Geometry: see drawing. Coordinates: mm, zero at the bounding-box minimum. A direction names the side the tool comes from. Coordinates: 2 decimals unless noted, no trailing zeros. Order: outer loops, then holes, each group sorted by start corner. A loop starts at its lowest first (then second) coordinate and runs counter-clockwise, first axis right, second up.
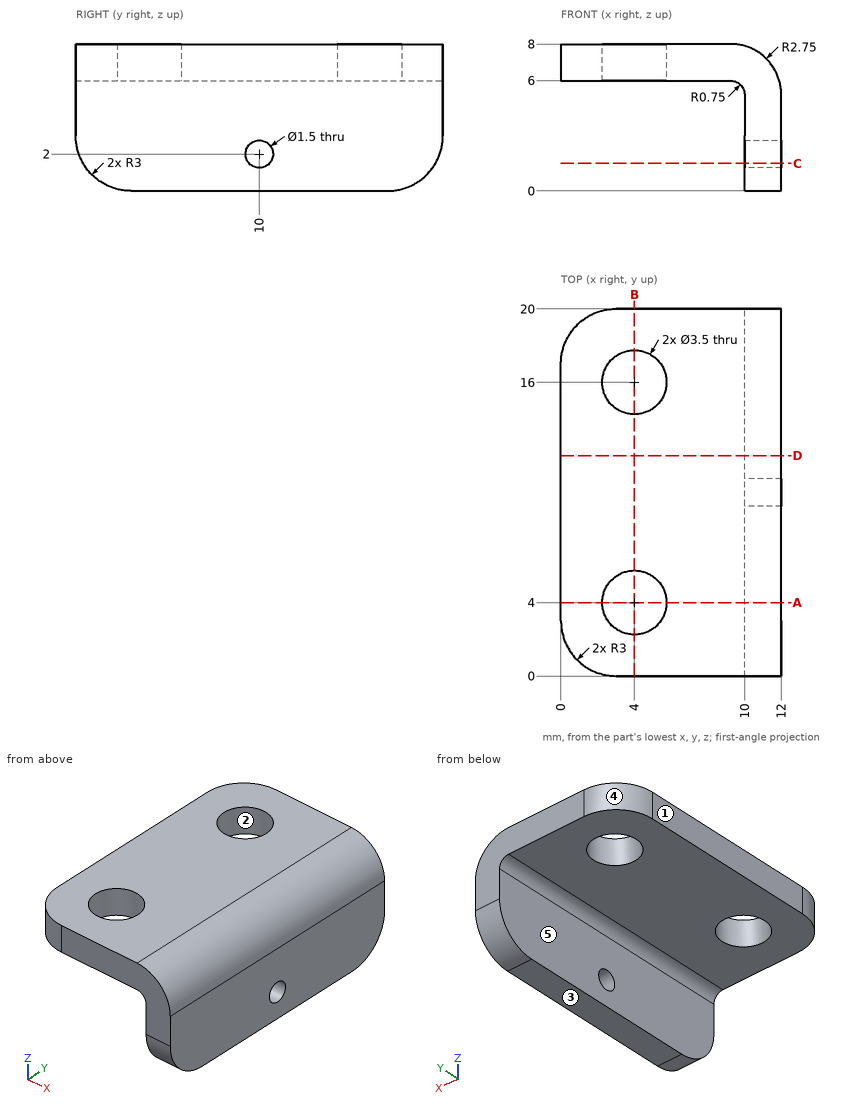
Item 1: Cut plane B-B on x = 4. Return loops of the section in (y, z).
Response values:
outline: (0, 6) - (2.25, 6) - (2.25, 8) - (0, 8) - close; (5.75, 6) - (14.25, 6) - (14.25, 8) - (5.75, 8) - close; (17.75, 6) - (20, 6) - (20, 8) - (17.75, 8) - close
Item 2: Access query for the marked faces 4 and 5. Directions: +Z, -Z, +X, -X, +Y, -Y. A direction counts if a zero-diameter tool reaches every point of the face in a straight line with its end or side. Return the directions, or none.
Response values:
face 4: +Z, -Z, -X, +Y
face 5: -Z, -X, +Y, -Y
Item 3: Cut plane A-A on y = 4. Return loops of the section in (x, z), then the cut area to 3 significant figures.
Response values:
outline: (0, 6) - (2.25, 6) - (2.25, 8) - (0, 8) - close; (5.75, 6) - (9.25, 6) arc R0.75 cw to (10, 5.25) - (10, 0) - (12, 0) - (12, 5.25) arc R2.75 ccw to (9.25, 8) - (5.75, 8) - close
area: 27.5 mm2
Item 4: Cut plane D-D on y = 12. Return loops of the section in (x, z), then the cut area to 3 significant figures.
Response values:
outline: (0, 6) - (9.25, 6) arc R0.75 cw to (10, 5.25) - (10, 0) - (12, 0) - (12, 5.25) arc R2.75 ccw to (9.25, 8) - (0, 8) - close
area: 34.5 mm2
Item 5: Draft query along X for the marked faces 1, 2 and 3. Return one class per face: pulls with the +X half, pulls with the -X half, needs draft (parallel to the pull), parting line crosses it, or undercut.
Response values:
face 1: pulls with the -X half
face 2: undercut
face 3: needs draft
Item 6: Ray query, probe 1 along Y at (x, z) = (4, 7.1); probe 2 along X at (y, z) = (3.5, 0.5); probe 3 along Z at (x, y) = (8, 15.5). Return the intervals inside material, ascending.
Response values:
probe 1: y = 0 to 2.25, 5.75 to 14.25, 17.75 to 20
probe 2: x = 10 to 12
probe 3: z = 6 to 8
Item 7: Cut plane C-C on z = 1.5. Return loops of the section in (x, y), then the cut area to 3 significant figures.
Response values:
outline: (10, 0.4) - (12, 0.4) - (12, 9.44) - (10, 9.44) - close; (10, 10.56) - (12, 10.56) - (12, 19.6) - (10, 19.6) - close
area: 36.2 mm2
Item 8: Pin query (flat end, axial travel): pin 1 Ø4.5 at (x, y) = (3, 11.5) entering from -Z; pin 2 Ø4 at (y, z) = (5.5, 1.5) entering from -X. Return the tip coordinate at first contact, or that it passes through.
Response values:
pin 1: stops at z = 6
pin 2: stops at x = 10
